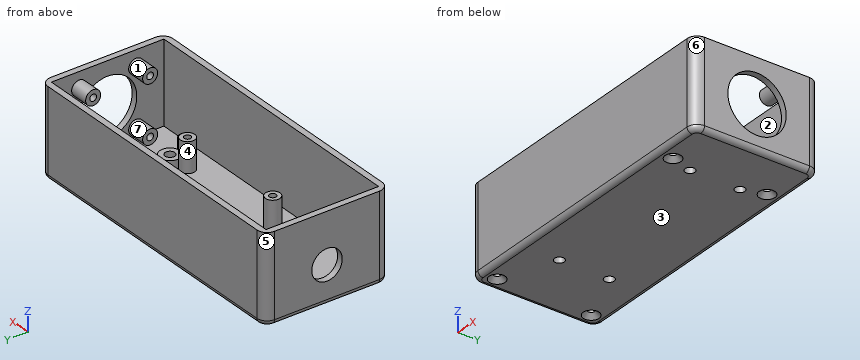
```python
from build123d import *

# Parameters (mm, degrees)
SKETCH_W            = 152.4
SKETCH_H            = 63.5
PAD_DEPTH           = 44.45
SKETCH001_W         = 146.05
SKETCH001_H         = 57.15
POCKET_DEPTH        = 41.275
SKETCH002_R         = 14.81709
POCKET001_DEPTH     = 5.0038
SKETCH003_R         = 3.81
PAD001_DEPTH        = 9.525
SKETCH004_R         = 1.7145
HOLE_DEPTH          = 10.16
HOLE_TIPS_R         = 1.7145
SKETCH005_R         = 7.747
POCKET002_DEPTH     = 25.4
SKETCH006_R         = 5.08
PAD002_DEPTH        = 7.62
SKETCH007_R         = 2.4765
HOLE001_DEPTH       = 24.9936
HOLE001_TIPS_R      = 2.4765
SKETCH008_R         = 3.81
PAD003_DEPTH        = 10.0076
HOLE002_D           = 3.4
HOLE002_DEPTH       = 126.5936
HOLE002_CSINK_D     = 8.0772
HOLE002_CSINK_ANGLE = 90
SKETCH010_R         = 3.683
PAD004_DEPTH        = 15.1384
SKETCH011_R         = 1.7145
HOLE003_DEPTH       = 10.16
HOLE003_TIPS_R      = 1.7145
SKETCH012_R         = 3.683
PAD005_DEPTH        = 10.7696
SKETCH013_R         = 1.7145
HOLE004_DEPTH       = 10.16
HOLE004_TIPS_R      = 1.7145
FILLET_R            = 5.08
FILLET001_R         = 2.54


with BuildPart() as part:
    # Sketch → Pad (new body)
    with BuildSketch(Plane.XY):
        Rectangle(SKETCH_W, SKETCH_H)
    extrude(amount=PAD_DEPTH)

    # Sketch001 → Pocket (cut)
    with BuildSketch(Plane.XY.offset(44.45)):
        Rectangle(SKETCH001_W, SKETCH001_H)
    extrude(amount=-POCKET_DEPTH, mode=Mode.SUBTRACT)

    # Sketch002 → Pocket001 (cut)
    with BuildSketch(Plane.YZ.offset(76.2)):
        with Locations((0, 22.2504)):
            Circle(SKETCH002_R)
    extrude(amount=-POCKET001_DEPTH, mode=Mode.SUBTRACT)

    # Sketch003 → Pad001 (join)
    with BuildSketch(Plane.YZ.offset(73.025)):
        with Locations((-14.478, 36.576)):
            Circle(SKETCH003_R)
        with Locations((14.478, 36.576)):
            Circle(SKETCH003_R)
        with Locations((14.478, 7.62)):
            Circle(SKETCH003_R)
        with Locations((-14.478, 7.62)):
            Circle(SKETCH003_R)
    extrude(amount=-PAD001_DEPTH)

    # Sketch004 → Hole (cut)
    with BuildSketch(Plane.YZ.offset(73.025)):
        with Locations((-14.478, 36.576)):
            Circle(SKETCH004_R)
        with Locations((14.478, 36.576)):
            Circle(SKETCH004_R)
        with Locations((14.478, 7.62)):
            Circle(SKETCH004_R)
        with Locations((-14.478, 7.62)):
            Circle(SKETCH004_R)
    extrude(amount=-HOLE_DEPTH, mode=Mode.SUBTRACT)

    # Hole tips → Hole tip 1 section 0
    with BuildSketch(Plane.YZ.offset(62.865), mode=Mode.PRIVATE) as hole_tip_1_s0:
        with Locations((-14.478, 36.576)):
            Circle(HOLE_TIPS_R)
    loft([hole_tip_1_s0.sketch, Vertex(61.834824, -14.478, 36.576)], mode=Mode.SUBTRACT)

    # Hole tips → Hole tip 2 section 0
    with BuildSketch(Plane.YZ.offset(62.865), mode=Mode.PRIVATE) as hole_tip_2_s0:
        with Locations((14.478, 36.576)):
            Circle(HOLE_TIPS_R)
    loft([hole_tip_2_s0.sketch, Vertex(61.834824, 14.478, 36.576)], mode=Mode.SUBTRACT)

    # Hole tips → Hole tip 3 section 0
    with BuildSketch(Plane.YZ.offset(62.865), mode=Mode.PRIVATE) as hole_tip_3_s0:
        with Locations((14.478, 7.62)):
            Circle(HOLE_TIPS_R)
    loft([hole_tip_3_s0.sketch, Vertex(61.834824, 14.478, 7.62)], mode=Mode.SUBTRACT)

    # Hole tips → Hole tip 4 section 0
    with BuildSketch(Plane.YZ.offset(62.865), mode=Mode.PRIVATE) as hole_tip_4_s0:
        with Locations((-14.478, 7.62)):
            Circle(HOLE_TIPS_R)
    loft([hole_tip_4_s0.sketch, Vertex(61.834824, -14.478, 7.62)], mode=Mode.SUBTRACT)

    # Sketch005 → Pocket002 (cut)
    with BuildSketch(Plane.YZ.offset(-76.2)):
        with Locations((0, 19.05)):
            Circle(SKETCH005_R)
    extrude(amount=POCKET002_DEPTH, mode=Mode.SUBTRACT)

    # Sketch006 → Pad002 (join)
    with BuildSketch(Plane.XY):
        with Locations((-41.275, 12.7)):
            Circle(SKETCH006_R)
        with Locations((47.625, 12.7)):
            Circle(SKETCH006_R)
        with Locations((47.625, -12.7)):
            Circle(SKETCH006_R)
        with Locations((-41.275, -12.7)):
            Circle(SKETCH006_R)
    extrude(amount=PAD002_DEPTH)

    # Sketch007 → Hole001 (cut)
    with BuildSketch(Plane.XY):
        with Locations((-41.275, 12.7)):
            Circle(SKETCH007_R)
        with Locations((47.625, 12.7)):
            Circle(SKETCH007_R)
        with Locations((47.625, -12.7)):
            Circle(SKETCH007_R)
        with Locations((-41.275, -12.7)):
            Circle(SKETCH007_R)
    extrude(amount=HOLE001_DEPTH, mode=Mode.SUBTRACT)

    # Hole001 tips → Hole001 tip 1 section 0
    with BuildSketch(Plane.XY.offset(24.9936), mode=Mode.PRIVATE) as hole001_tip_1_s0:
        with Locations((-41.275, 12.7)):
            Circle(HOLE001_TIPS_R)
    loft([hole001_tip_1_s0.sketch, Vertex(-41.275, 12.7, 26.481631)], mode=Mode.SUBTRACT)

    # Hole001 tips → Hole001 tip 2 section 0
    with BuildSketch(Plane.XY.offset(24.9936), mode=Mode.PRIVATE) as hole001_tip_2_s0:
        with Locations((47.625, 12.7)):
            Circle(HOLE001_TIPS_R)
    loft([hole001_tip_2_s0.sketch, Vertex(47.625, 12.7, 26.481631)], mode=Mode.SUBTRACT)

    # Hole001 tips → Hole001 tip 3 section 0
    with BuildSketch(Plane.XY.offset(24.9936), mode=Mode.PRIVATE) as hole001_tip_3_s0:
        with Locations((47.625, -12.7)):
            Circle(HOLE001_TIPS_R)
    loft([hole001_tip_3_s0.sketch, Vertex(47.625, -12.7, 26.481631)], mode=Mode.SUBTRACT)

    # Hole001 tips → Hole001 tip 4 section 0
    with BuildSketch(Plane.XY.offset(24.9936), mode=Mode.PRIVATE) as hole001_tip_4_s0:
        with Locations((-41.275, -12.7)):
            Circle(HOLE001_TIPS_R)
    loft([hole001_tip_4_s0.sketch, Vertex(-41.275, -12.7, 26.481631)], mode=Mode.SUBTRACT)

    # Sketch008 → Pad003 (join)
    with BuildSketch(Plane.XY):
        with Locations((-68.58, 23.876)):
            Circle(SKETCH008_R)
        with Locations((-68.58, -23.876)):
            Circle(SKETCH008_R)
        with Locations((51.054, 23.876)):
            Circle(SKETCH008_R)
        with Locations((51.054, -23.876)):
            Circle(SKETCH008_R)
    extrude(amount=PAD003_DEPTH)

    # Hole002
    with Locations(Plane(origin=(0, 0, 0), x_dir=(1, 0, 0), z_dir=(0, 0, -1))):
        with Locations((-68.58, -23.876), (-68.58, 23.876), (51.054, -23.876), (51.054, 23.876)):
            CounterSinkHole(HOLE002_D / 2, HOLE002_CSINK_D / 2, depth=HOLE002_DEPTH, counter_sink_angle=HOLE002_CSINK_ANGLE)

    # Sketch010 → Pad004 (join)
    with BuildSketch(Plane.XY.offset(3.175)):
        with Locations((-18.034, 7.1374)):
            Circle(SKETCH010_R)
        with Locations((-18.034, -15.875)):
            Circle(SKETCH010_R)
        with Locations((39.9542, -15.875)):
            Circle(SKETCH010_R)
    extrude(amount=PAD004_DEPTH)

    # Sketch011 → Hole003 (cut)
    with BuildSketch(Plane.XY.offset(18.3134)):
        with Locations((-18.034, 7.1374)):
            Circle(SKETCH011_R)
        with Locations((-18.034, -15.875)):
            Circle(SKETCH011_R)
        with Locations((39.9542, -15.875)):
            Circle(SKETCH011_R)
    extrude(amount=-HOLE003_DEPTH, mode=Mode.SUBTRACT)

    # Hole003 tips → Hole003 tip 1 section 0
    with BuildSketch(Plane.XY.offset(8.1534), mode=Mode.PRIVATE) as hole003_tip_1_s0:
        with Locations((-18.034, 7.1374)):
            Circle(HOLE003_TIPS_R)
    loft([hole003_tip_1_s0.sketch, Vertex(-18.034, 7.1374, 7.123224)], mode=Mode.SUBTRACT)

    # Hole003 tips → Hole003 tip 2 section 0
    with BuildSketch(Plane.XY.offset(8.1534), mode=Mode.PRIVATE) as hole003_tip_2_s0:
        with Locations((-18.034, -15.875)):
            Circle(HOLE003_TIPS_R)
    loft([hole003_tip_2_s0.sketch, Vertex(-18.034, -15.875, 7.123224)], mode=Mode.SUBTRACT)

    # Hole003 tips → Hole003 tip 3 section 0
    with BuildSketch(Plane.XY.offset(8.1534), mode=Mode.PRIVATE) as hole003_tip_3_s0:
        with Locations((39.9542, -15.875)):
            Circle(HOLE003_TIPS_R)
    loft([hole003_tip_3_s0.sketch, Vertex(39.9542, -15.875, 7.123224)], mode=Mode.SUBTRACT)

    # Sketch012 → Pad005 (join)
    with BuildSketch(Plane.XY.offset(3.175)):
        with Locations((39.9542, 7.1374)):
            Circle(SKETCH012_R)
    extrude(amount=PAD005_DEPTH)

    # Sketch013 → Hole004 (cut)
    with BuildSketch(Plane.XY.offset(13.9446)):
        with Locations((39.9542, 7.1374)):
            Circle(SKETCH013_R)
    extrude(amount=-HOLE004_DEPTH, mode=Mode.SUBTRACT)

    # Hole004 tips → Hole004 tip 1 section 0
    with BuildSketch(Plane.XY.offset(3.7846), mode=Mode.PRIVATE) as hole004_tip_1_s0:
        with Locations((39.9542, 7.1374)):
            Circle(HOLE004_TIPS_R)
    loft([hole004_tip_1_s0.sketch, Vertex(39.9542, 7.1374, 2.754424)], mode=Mode.SUBTRACT)

    # Fillet
    fillet_edges = [part.edges().sort_by_distance(p)[0] for p in [
        (76.2, 31.75, 22.225),
        (-76.2, 31.75, 22.225),
        (-76.2, -31.75, 22.225),
        (76.2, -31.75, 22.225),
    ]]
    fillet(fillet_edges, radius=FILLET_R)

    # Fillet001
    fillet001_edges = [part.edges().sort_by_distance(p)[0] for p in [
        (0, -31.75, 0),
    ]]
    fillet(fillet001_edges, radius=FILLET001_R)


solid = part.part
```
Design review of the part built by this model. Coordinates are the model's own, in mm. Face numbers are marked on the shaded views. A direction names the side the tool comes from. Round coordinates to 2 decimals unless told otherwise and drop trailing zeros. Order: outer loops, then holes, each group sorted by start corner. A loop starts at its lowest first (then second) coordinate and runs counter-clockwise, first axis right, second up. Notation, with made-up numbers: (-32, 61) - (11, 61) arc R22 cw to (11, 78) - close; hole circle Ø4 at (74.25, 51). An arc over 180 degrees is marked (long way). Return JSON: item names as keys, results as strings.
Q1. Consider section C-C on z = 25. Write out the cut boundary in (x, y) (3 decimals), plus the area to 3 significant figures.
Computed values:
{"outline": "(-76.2, -26.67) arc R5.08 ccw to (-71.12, -31.75) - (71.12, -31.75) arc R5.08 ccw to (76.2, -26.67) - (76.2, -14.56) - (73.025, -14.56) - (73.025, -28.575) - (-73.025, -28.575) - (-73.025, -4.961) - (-76.2, -4.961) - close; (-76.2, 4.961) - (-73.025, 4.961) - (-73.025, 28.575) - (73.025, 28.575) - (73.025, 14.56) - (76.2, 14.56) - (76.2, 26.67) arc R5.08 ccw to (71.12, 31.75) - (-71.12, 31.75) arc R5.08 ccw to (-76.2, 26.67) - close", "area": "1,180 mm2"}
Q2. Machinability: for the marked faces 1, 2 and 3, which of the approach directions +Z, -Z, +X, -X, +Y, -Y give a long, thin tool a straight path to every point of the face, cutting with its end or side? Answer none if there is none.
Computed values:
{"face 1": "none", "face 2": "+Z", "face 3": "-Z, +X, -X, +Y, -Y"}
Q3. Consider section D-D on x = -2.5. Write out the cut boundary in (y, z) (3 decimals), plus the area to 3 significant figures.
Computed values:
{"outline": "(-31.75, 2.54) arc R2.54 ccw to (-29.21, 0) - (29.21, 0) arc R2.54 ccw to (31.75, 2.54) - (31.75, 44.45) - (28.575, 44.45) - (28.575, 3.175) - (-28.575, 3.175) - (-28.575, 44.45) - (-31.75, 44.45) - close", "area": "461 mm2"}
Q4. Consider section B-B on y = 0. Write out the cut boundary in (x, z) (3 decimals).
Computed values:
{"outline": "(-76.2, 2.54) arc R2.54 ccw to (-73.66, 0) - (73.66, 0) arc R2.54 ccw to (76.2, 2.54) - (76.2, 7.433) - (73.025, 7.433) - (73.025, 3.175) - (-73.025, 3.175) - (-73.025, 11.303) - (-76.2, 11.303) - close; (-76.2, 26.797) - (-73.025, 26.797) - (-73.025, 44.45) - (-76.2, 44.45) - close; (73.025, 37.067) - (76.2, 37.067) - (76.2, 44.45) - (73.025, 44.45) - close"}
Q5. Consider section A-A on x = -68.58. Give the number of separate pieces and of enclosed holes in the cut face, plus the area to 3 significant figures.
Computed values:
{"separate pieces": "3", "enclosed holes": "0", "area": "486 mm2"}
Q6. For pin 1 Ø6 at (x, y) = (52.5, 25.5) entering from +Z; pin 2 Ø2.5 at (x, y) = (-68.58, -23.876) entering from +Z; pin 3 Ø2 at (x, y) = (31, -9.5) entering from +Z (3 decimals); pin 4 Ø2.5 at (x, y) = (-18.034, -15.875) entering from -Z, all flat-tipped, find the tip position at first contact; note any pin that passes through.
Computed values:
{"pin 1": "stops at z = 10.01", "pin 2": "passes through", "pin 3": "stops at z = 3.175", "pin 4": "stops at z = 0"}
Q7. Wall thickness on L1, parallel to Y at x = -53.5, z = 27.5 (3 decimals); L2, parallel to X at y = -4.5, z = 5 (3 decimals); L3, parallel to X at y = 12, z = 3: over which ranges is each line inside the solid? List them lowest first. Write a range as [from, to].
Computed values:
{"L1": "y = [-31.75, -28.575], [28.575, 31.75]", "L2": "x = [-76.2, -73.025], [73.025, 76.2]", "L3": "x = [-76.2, -43.65], [-38.9, 45.25], [50, 76.2]"}
Q8. The part is to be moulded in two halves that separate along X. For the marked faces 4, 5, 6 and 7, say which applies: pulls with the +X half, pulls with the -X half, needs draft (parallel to the pull), parting line crosses it, or undercut.
Computed values:
{"face 4": "undercut", "face 5": "pulls with the -X half", "face 6": "pulls with the +X half", "face 7": "undercut"}
